Work out the finished part from the listing and answer in its coordinate system (mm). Face numbers are marked on the shaded views. A direction names the side the tool comes from. Round coordinates to 2 decimals unless told otherwise and drop trailing zeros. Write each loop counter-clockwise with the first axis right and the second up, starting at its lowest first coordinate (ties: lowest second). Pieces come first, ordered by that corner, then holes.
1. A tool of negligible diameter and unlimited length cuts with its end or side. For the marked faces 1, 2 and 3, from which of +Z, -Z, +X, -X, +Y, -Y can it reach the whole face along a straight path? Write none if from no direction.
2. Straight lines are drawn through the part: probe 1 along Y at (x, z) = (0, 1.4); probe 2 along Z at (x, y) = (-5.75, 3.75); probe 3 along Y at (x, z) = (8, 0.55). For each, find the intervals that lie inside material, in ascending order.
3. Find section C-C (x = -8). Write down the section's boundary in (y, z).
4. Flat-ended cylindrical pins translate along their axes: pin 1 Ø0.9 at (y, z) = (0.5, 16) entering from +X; pin 2 Ø5 at (x, z) = (-4, 10) entering from -Y; pin 3 Ø5 at (x, y) = (2.5, -6.5) entering from +Z. Find the tip coordinate at first contact, or state that the pin passes through.
5. Find section A-A (x = 0). Write down the section's boundary in (y, z), and give its area (3 significant figures).
6. Find section B-B (y = 0). Write down the section's boundary in (x, z).
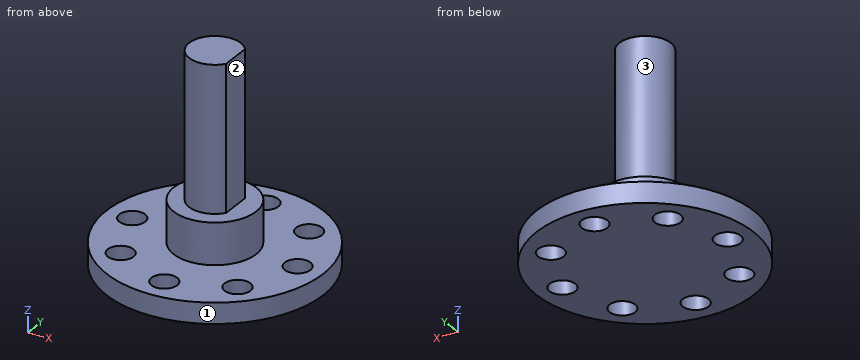
Autodesk Inventor part; units mm, degrees
ref_plane "YZ Plane" through (0, 0, 0) normal (1, 0, 0) x (0, 1, 0)
ref_plane "XZ Plane" through (0, 0, 0) normal (0, 1, 0) x (-1, 0, 0)
ref_plane "XY Plane" through (0, 0, 0) normal (0, 0, 1) x (1, 0, 0)
sketch "Sketch1" plane through (0, 0, 0) normal (0, 0, 1) x (1, 0, 0)
  circle A0 centre (0, 0) radius 10.5
  line L0 (0, 0) -> (8, 0)
  circle A1 centre (8, 0) radius 1.25
  circle A2 centre (5.6569, 5.6569) radius 1.25
  circle A3 centre (0, 8) radius 1.25
  circle A4 centre (-5.6569, 5.6569) radius 1.25
  circle A5 centre (-8, 0) radius 1.25
  circle A6 centre (-5.6569, -5.6569) radius 1.25
  circle A7 centre (0, -8) radius 1.25
  circle A8 centre (5.6569, -5.6569) radius 1.25
  dimension "d0" = 21
  dimension "d1" = 8
  dimension "d2" = 2.5
  dimension "d5" = 360
extrude "Extrusion1" add sketch "Sketch1" along normal blind 2
sketch "Sketch2" plane through (0, 0, 2) normal (0, 0, 1) x (1, 0, 0)
  circle A0 centre (0, 0) radius 2.5
  dimension "d9" = 5
extrude "Extrusion3" add sketch "Sketch2" along normal blind 18
sketch "Sketch3" plane through (0, 0, 2) normal (0, 0, 1) x (1, 0, 0)
  circle A0 centre (0, 0) radius 2.5
  circle A1 centre (0, 0) radius 4
  dimension "d14" = 8
extrude "Extrusion4" add sketch "Sketch3" along normal blind 4
sketch "Sketch4" plane through (0, 0, 20) normal (0, 0, 1) x (1, 0, 0)
  line L0 (0, 0) -> (2, 0)
  line L1 (0, 0) -> (2, 0) construction
  line L2 (2, 0) -> (2, 1.5)
  circle A0 centre (0, 0) radius 2.5
  line L3 (2, 0) -> (2, -1.5)
  circle A1 centre (0, 0) radius 2.5
  dimension "d17" = 2
  dimension "d18" = 0
extrude "Extrusion5" cut sketch "Sketch4" against normal blind 14 contours L2 A0 L3 picked at (2.0912, -0.8466)
properties part number "Drive_shaft"
Worked answers:
1. face 1: +Z, -Z
1. face 2: +Z, +X, +Y, -Y
1. face 3: +Z
2. probe 1: y = -10.5 to -9.25, -6.75 to 6.75, 9.25 to 10.5
2. probe 2: z = 0 to 2
2. probe 3: y = -6.8 to -1.25, 1.25 to 6.8
3. outline: (-6.8, 0) - (-1.25, 0) - (-1.25, 2) - (-6.8, 2) - close; (1.25, 0) - (6.8, 0) - (6.8, 2) - (1.25, 2) - close
4. pin 1: stops at x = 2
4. pin 2: stops at y = -2
4. pin 3: stops at z = 2
5. outline: (-10.5, 0) - (-9.25, 0) - (-9.25, 2) - (-10.5, 2) - close; (-6.75, 0) - (6.75, 0) - (6.75, 2) - (4, 2) - (4, 6) - (2.5, 6) - (2.5, 20) - (-2.5, 20) - (-2.5, 6) - (-4, 6) - (-4, 2) - (-6.75, 2) - close; (9.25, 0) - (10.5, 0) - (10.5, 2) - (9.25, 2) - close
5. area: 134 mm2
6. outline: (-10.5, 0) - (-9.25, 0) - (-9.25, 2) - (-10.5, 2) - close; (-6.75, 0) - (6.75, 0) - (6.75, 2) - (4, 2) - (4, 6) - (2, 6) - (2, 20) - (-2.5, 20) - (-2.5, 6) - (-4, 6) - (-4, 2) - (-6.75, 2) - close; (9.25, 0) - (10.5, 0) - (10.5, 2) - (9.25, 2) - close
